Geometry check sheet. Reference: the model listing, model coordinates, mm. A direction names the side the tool comes from. Coordinates: 2 decimals unless noted, no trailing zeros. Order: outer loops, then holes, each group sorted by start corner. A loop starts at its lowest first (then second) coordinate and runs counter-clockwise, first axis right, second up. Notation, with made-up numbers: M 80,-26 L 130,-26 A5 ccw 130,-21 Z; hole C 11.5,-34 d9. An arc over 180 degrees is marked long. One line per item, written item: value. Start each with the question number.
1) Access from +Z, -Z, +X, -X, +Y, -Y to the whole of each face (thin tool, end or side, straight path). Record for faces 1 (the flat face through (0.3, 0.4, 0)), 2 (the flat face through (3, 3, 0)), 3 (the flat face through (8, 2, 9.525)), 4 (the flat face through (2.8, 0.3, 0)).
2) Sectioned sample at A-A, the plane z = 7. Enter the section's corners in (x, y) (3 decimals).
3) Go/stop test with flat-tipped pins: P1, Ø1.5, axis at x = 12, z = 1, coming from the -Y side; P2, Ø1.6, axis at x = 14, y = 1, coming from the -Z side (3 decimals). Record where each tip stops, or that it passes through.
4) Thickness scan on L1, parallel to X at y = 2.05, z = 4 (3 decimals); L2, parallel to Z at x = 13.75, y = 2.6 (3 decimals); L3, parallel to Z at x = 7, y = 2.3 (3 decimals). Record the ranges inside material, lowest first. Write a range as from..to.
5) Sectioned sample at C-C, the plane x = 13. Enter the section's corners in (y, z) (3 decimals).
6) Draft check along X on faces 5 (the cylindrical face through (1.38, 3.16, -3.13)), 6 (the flat face through (0.3, 2.8, 0)), 7 (the flat face through (3.175, 2, 5)). Enter one of: pulls with the +X half, pulls with the -X half, needs draft (parallel to the pull), parting line crosses it, or undercut.
7) Sectioned sample at D-D, the plane z = -2.5. Enter the section's corners in (x, y) (1 decimal).
8) Sectioned sample at B-B, the plane y = 0.7. Enter the section's corners in (x, z) (3 decimals), then the cut area to 3 significant figures.
```python
from build123d import *

# Parameters (mm, degrees)
F0_W     = 3.175
F0_H     = 3.175
F1_DEPTH = 12.7
F2_W     = 3.175
F2_H     = 3.175
F3_DEPTH = 12.7
F4_W     = 3.175
F4_H     = 3.175
F5_DEPTH = 6.35
F6_R     = 1.5875
F7_DEPTH = 6.35


with BuildPart() as f1:
    # F0 (on Top) → F1 (new body)
    with BuildSketch(Plane.XY):
        with Locations((1.5875, 1.5875)):
            Rectangle(F0_W, F0_H)
    extrude(amount=F1_DEPTH)

    # F2 (on face) → F3 (join)
    with BuildSketch(Plane.YZ.offset(3.175)):
        with Locations((1.5875, 11.1125)):
            Rectangle(F2_W, F2_H)
    extrude(amount=F3_DEPTH)

    # F4 (on face) → F5 (join)
    with BuildSketch(Plane(origin=(0, 0, 9.525), x_dir=(1, 0, 0), z_dir=(0, 0, -1))):
        with Locations((14.2875, -1.5875)):
            Rectangle(F4_W, F4_H)
    extrude(amount=F5_DEPTH)

    # F6 (on Top) → F7 (join)
    with BuildSketch(Plane.XY):
        with Locations((1.5875, 1.5875)):
            Circle(F6_R)
    extrude(amount=-F7_DEPTH)


solid = f1.part
```
Final values:
1. face 1: -Z, -X, -Y
1. face 2: -Z, +X, +Y
1. face 3: -Z, +Y, -Y
1. face 4: -Z, +X, -Y
2. outline: M 0,0 L 3.175,0 L 3.175,3.175 L 0,3.175 Z; M 12.7,0 L 15.875,0 L 15.875,3.175 L 12.7,3.175 Z
3. P1: passes through
3. P2: stops at z = 3.175
4. L1: x = 0..3.175, 12.7..15.875
4. L2: z = 3.175..12.7
4. L3: z = 9.525..12.7
5. outline: M 0,3.175 L 3.175,3.175 L 3.175,12.7 L 0,12.7 Z
6. face 5: parting line crosses it
6. face 6: needs draft
6. face 7: undercut
7. outline: C 1.6,1.6 d3.2
8. outline: M 0,0 L 0.271,0 L 0.271,-6.35 L 2.904,-6.35 L 2.904,0 L 3.175,0 L 3.175,9.525 L 12.7,9.525 L 12.7,3.175 L 15.875,3.175 L 15.875,12.7 L 0,12.7 Z
8. area: 118 mm^2
